Autodesk Inventor part; units mm, degrees
ref_plane "Pracovní rovina1" through (-3, 0, 102) normal (1, 0, 0) x (0, 0, -1)
ref_plane "YZ Plane" through (0, 0, 0) normal (1, 0, 0) x (0, 1, 0)
ref_plane "XZ Plane" through (0, 0, 0) normal (0, 1, 0) x (-1, 0, 0)
sketch "Náčrt1" plane through (0, 0, 0) normal (0, 0, 1) x (1, 0, 0)
  circle A0 centre (0, 0) radius 1
  dimension "d0" = 2
extrude "Vysunutí1" add sketch "Náčrt1" along normal blind 100
sketch "Náčrt2" plane through (0, 0, 100) normal (0, 0, 1) x (1, 0, 0)
  line L0 (-5, 1) -> (5, 1)
  line L1 (5, 1) -> (5, -1)
  line L2 (5, -1) -> (-5, -1)
  line L3 (-5, -1) -> (-5, 1)
  line L4 (-7, 0) -> (7, 0)
  line L5 (0, 1.4) -> (0, -1.4)
  point P0 (0, 0)
  dimension "d3" = 10
extrude "Vysunutí2" add sketch "Náčrt2" along normal blind 2
sketch "Náčrt3" plane through (0, 0, 102) normal (0, 0, 1) x (1, 0, 0)
  line L0 (-5, -1) -> (5, -1)
  line L1 (5, -1) -> (5, 1)
  line L2 (5, 1) -> (-5, 1)
  line L3 (-5, 1) -> (-5, -1)
  circle A0 centre (-4, 0) radius 1
  circle A1 centre (4, 0) radius 1
  point P0 (0, 0)
extrude "Vysunutí3" add sketch "Náčrt3" along normal blind 10 contours A0 | A1
ref_plane "Pracovní rovina1" through (-3, 0, 102) normal (1, 0, 0) x (0, 0, -1)
sketch "Náčrt4" plane through (-3, 0, 102) normal (1, 0, 0) x (0, 0, -1)
  line L0 (-10, 1) -> (-10, -1)
  line L1 (0, 1) -> (0, -1)
  line L2 (0, 0) -> (0, 1)
  line L3 (0, -1) -> (0, 0)
  line L4 (0, 1) -> (-10, 1)
  line L5 (0, -1) -> (-10, -1)
  circle A0 centre (-9, 0) radius 1
  point P0 (102, 0)
extrude "Vysunutí4" add sketch "Náčrt4" along normal blind 8 and the other way blind 2 contours A0
properties part number "táhlo"
Verification items for the finished model (mm, model axes). A direction names the side the tool comes from. Give positions to 0.01 mm unless a question says otherwise; leave off trailing zeros. Loops run counter-clockwise (first coordinate to the right, second up) from the corner with the lowest first, then second, coordinate; pieces in that order, holes last.
1. Section check B-B, the plane y = -0.55. Enter the section's corners in (x, z).
2. Thickness scan on line 1 (Z direction, x = 2.25, y = 0); line 2 (Z direction, x = -0.75, y = 0); line 3 (X direction, y = 0.2, z = 17). Record the ranges inside material, lowest first.
3. Section check A-A, the plane z = 104. Enter the section's corners in (x, y), then the cut area to 3 significant figures.
4. Go/stop test with flat-tipped pins: pin 1 Ø0.6 at (x, y) = (-1, 0.5) entering from +Z; pin 2 Ø1 at (x, z) = (2.5, 79.5) entering from +Y; pin 3 Ø1 at (y, z) = (0, 88.5) entering from +X; pin 4 Ø6 at (x, z) = (-3, 70.5) entering from +Y. Record where each tip stops, or that it passes through.
5. Section check C-C, the plane z = 68.5. Enter the section's corners in (x, y), then the cut area to 3 significant figures.
6. Set-up check for faces 1 (the flat face through (-4, 0, 112)), 2 (the cylindrical face through (0, 1, 49)), 3 (the cylindrical face through (-3, 0, 106)): record each of +Z, -Z, +X, -X, +Y, -Y from which the full face is reachable in a straight line by a thin tool's end or side.
Geometry says:
1. outline: (-5, 100) - (-0.84, 100) - (-0.84, 0) - (0.84, 0) - (0.84, 100) - (5, 100) - (5, 102) - (4.84, 102) - (4.84, 110.16) - (5, 110.16) - (5, 111.84) - (4.84, 111.84) - (4.84, 112) - (3.16, 112) - (3.16, 111.84) - (-3.16, 111.84) - (-3.16, 112) - (-4.84, 112) - (-4.84, 111.84) - (-5, 111.84) - (-5, 110.16) - (-4.84, 110.16) - (-4.84, 102) - (-5, 102) - close; hole (-3.16, 102) - (3.16, 102) - (3.16, 110.16) - (-3.16, 110.16) - close
2. line 1: z = 100 to 102, 110 to 112
2. line 2: z = 0 to 102, 110 to 112
2. line 3: x = -0.98 to 0.98
3. outline: circle Ø2 at (-4, 0); circle Ø2 at (4, 0)
3. area: 6.28 mm2
4. pin 1: stops at z = 111.98
4. pin 2: passes through
4. pin 3: stops at x = 1
4. pin 4: stops at y = 1
5. outline: circle Ø2 at (0, 0)
5. area: 3.14 mm2
6. face 1: +Z, +X, -X, +Y, -Y
6. face 2: -Z
6. face 3: none
